Input: part model. Units: mm. Frame: model coordinates. Coordinates: 2 decimals unless noted, no trailing zeros. Order: outer loops, then holes, each group sorted by start corner. A loop starts at its lowest first (then second) coordinate and runs counter-clockwise, first axis right, second up. Notation, with made-up numbers: (10, 29) -> (22, 29) arc R21 ccw to (22, 36) -> close; hole circle Ø9 at (84, -27). An arc over 180 degrees is marked (long way). Answer as CSV lines item,"result".
from build123d import *

# Parameters (mm, degrees)
ESQUISSE1_R        = 8
ESQUISSE1_R_2      = 4.55
BOSS_EXTRU_1_DEPTH = 16.5
CHANFREIN1_SIZE    = 0.3


with BuildPart() as part:
    # Esquisse1 → Boss.-Extru.1 (new body)
    with BuildSketch(Plane(origin=(0, 0, 0), x_dir=(1, 0, 0), z_dir=(0, 1, 0))):
        with Locations(Location((0, 0, 0), (0, 0, 270))):
            Circle(ESQUISSE1_R)
        with Locations(Location((0, 0, 0), (0, 0, 270))):
            Circle(ESQUISSE1_R_2, mode=Mode.SUBTRACT)
    extrude(amount=BOSS_EXTRU_1_DEPTH)

    # Chanfrein1
    chanfrein1_edges = [part.edges().sort_by_distance(p)[0] for p in [
        (0, 0, -8),
        (0, 16.5, -8),
        (0, 0, -4.55),
        (0, 16.5, -4.55),
    ]]
    chamfer(chanfrein1_edges, length=CHANFREIN1_SIZE)


solid = part.part
1. Cut plane C-C (y = 3.25). Return the cut outline in (x, z).
Findings:
outline,"circle Ø16 at (0, 0); hole circle Ø9.1 at (0, 0)"
2. Ray query, line 1 along X through (y, z) = (9.25, 0); line 2 along Z through (x, y) = (1.5, 10.25); line 3 along X through (y, z) = (6.5, -3.25). Return the intervals inside material, ascending.
Findings:
line 1,"x = -8 to -4.55, 4.55 to 8"
line 2,"z = -7.86 to -4.3, 4.3 to 7.86"
line 3,"x = -7.31 to -3.18, 3.18 to 7.31"
3. Contact query for flat-ended pins moving along their axis: pin 1 (6 mm diameter, centred on y = 7.5, z = 4, fed in from +X); pin 2 (5 mm diameter, centred on x = -5, y = 10, fed in from -Z); pin 3 (2 mm diameter, centred on x = 3, z = 2, fed in from -Y). Output: stop coordinate, or through.
Findings:
pin 1,"stops at x = 7.94"
pin 2,"stops at z = -7.6"
pin 3,"stops at y = 0.24"
4. Cut plane A-A (x = 0). Return the cut outline in (y, z).
Findings:
outline,"(0, -7.7) -> (0.3, -8) -> (16.2, -8) -> (16.5, -7.7) -> (16.5, -4.85) -> (16.2, -4.55) -> (0.3, -4.55) -> (0, -4.85) -> close; (0, 4.85) -> (0.3, 4.55) -> (16.2, 4.55) -> (16.5, 4.85) -> (16.5, 7.7) -> (16.2, 8) -> (0.3, 8) -> (0, 7.7) -> close"
5. Mould query, pull axis X, two halves, no side actions, for faces 1 (the face through (-7.81, 8.14, -1.73)), 2 (the face through (-5, 0, 0)), 3 (the face through (-2.77, 8.14, -3.61)). Classes: released by +X, released by -X, zero draft, split by the parting line, or undercut.
Findings:
face 1,"split by the parting line"
face 2,"zero draft"
face 3,"undercut"
6. Cut plane B-B (z = 0). Return the cut outline in (x, y).
Findings:
outline,"(-8, 0.3) -> (-7.7, 0) -> (-4.85, 0) -> (-4.55, 0.3) -> (-4.55, 16.2) -> (-4.85, 16.5) -> (-7.7, 16.5) -> (-8, 16.2) -> close; (4.55, 0.3) -> (4.85, 0) -> (7.7, 0) -> (8, 0.3) -> (8, 16.2) -> (7.7, 16.5) -> (4.85, 16.5) -> (4.55, 16.2) -> close"
